```python
from build123d import *

# Parameters (mm, degrees)
SKETCH1_W           = 43.67
SKETCH1_H           = 21.69
SKETCH1_R           = 1.5
BOSS_EXTRUDE1_DEPTH = 1.5
SKETCH2_W           = 2.5
SKETCH2_H           = 2.5
BOSS_EXTRUDE2_DEPTH = 0.01
SKETCH3_W           = 2.5
SKETCH3_H           = 2.5
BOSS_EXTRUDE3_DEPTH = 0.01
SKETCH4_R           = 5
BOSS_EXTRUDE4_DEPTH = 12


with BuildPart() as part:
    # Sketch1 → Boss-Extrude1 (new body)
    with BuildSketch(Plane(origin=(0, 0, 0), x_dir=(1, 0, 0), z_dir=(0, 1, 0))):
        Rectangle(SKETCH1_W, SKETCH1_H)
        with Locations(Location((-15.145, 8.035, 0), (0, 0, 270))):
            Circle(SKETCH1_R, mode=Mode.SUBTRACT)
        with Locations(Location((15.095, -8.345, 0), (0, 0, 270))):
            Circle(SKETCH1_R, mode=Mode.SUBTRACT)
    extrude(amount=BOSS_EXTRUDE1_DEPTH)

    # Sketch2 → Boss-Extrude2 (add)
    with BuildSketch(Plane(origin=(0, 1.5, 0), x_dir=(1, 0, 0), z_dir=(0, 1, 0))):
        with Locations((-20.585, 9.595)):
            Rectangle(SKETCH2_W, SKETCH2_H)
        with Locations((-20.585, -9.595)):
            Rectangle(SKETCH2_W, SKETCH2_H)
    extrude(amount=BOSS_EXTRUDE2_DEPTH)

    # Sketch3 → Boss-Extrude3 (add)
    with BuildSketch(Plane(origin=(0, 1.5, 0), x_dir=(1, 0, 0), z_dir=(0, 1, 0))):
        with Locations((20.585, 9.595)):
            Rectangle(SKETCH3_W, SKETCH3_H)
        with Locations((20.585, -9.595)):
            Rectangle(SKETCH3_W, SKETCH3_H)
    extrude(amount=BOSS_EXTRUDE3_DEPTH)

    # Sketch4 → Boss-Extrude4 (add)
    with BuildSketch(Plane(origin=(0, 1.5, 0), x_dir=(1, 0, 0), z_dir=(0, 1, 0))):
        with Locations(Location((-12, 0, 0), (0, 0, 90))):
            Circle(SKETCH4_R)
        with Locations(Location((12, 0, 0), (0, 0, 90))):
            Circle(SKETCH4_R)
    extrude(amount=BOSS_EXTRUDE4_DEPTH)


solid = part.part
```
The listing builds one solid part. Answer for the finished solid, in the listing's coordinates (mm). A direction names the side the tool comes from. Coordinates: 2 decimals unless noted, no trailing zeros. Loops run counter-clockwise (first coordinate to the right, second up) from the corner with the lowest first, then second, coordinate; pieces in that order, holes last. Notation, with made-up numbers: M -35.5,21.5 L -28.5,21.5 A25 ccw -28.5,57.5 Z; hole C 87,76.5 d11. An arc over 180 degrees is marked long. Answer as a JSON object with one key per item and string values. Group by question number.
Item 1: Section C-C (y = 10.5) is taken. Write down the section's boundary in (x, z).
Item 2: Consider L1, parallel to Y at x = 11.5, z = 5.25; L2, parallel to X at y = 5.5, z = 2; L3, parallel to X at y = 1.75, z = 1.5. Determine where each line is inside the solid, lowest interval first.
Item 3: Section B-B (x = 12) is taken. Write down the section's boundary in (y, z) (3 decimals), and give its area (3 significant figures).
Item 4: Section A-A (z = 0) is taken. Write down the section's boundary in (x, y) (3 decimals), and give its area (3 significant figures).
Item 5: Which of the six approach directions +Z, -Z, +X, -X, +Y, -Y give full straight-line access (tool end or side, diameter ignored) to faces 4 (the face through (-21, 1.51, -10)), 5 (the face through (8, 7, -3))?
Item 6: Section D-D (x = 3) is taken. Write down the section's boundary in (y, z) (3 decimals).
Item 7: Determine the mould class of faces 1 (the face through (15.546, 0.74, 9.776)), 2 (the face through (-21.835, 1, 0)), 3 (the face through (21, 1.51, 10)) for opening direction X: +X half, -X half, draft (parallel to the pull), parting line (faces both ways), or undercut.
Item 8: Each of these flat-tipped pins is pushed along its axis until it touches: P1, Ø3, axis at x = -20, z = -10, coming from the +Y side; P2, Ø1.8, axis at x = 15.095, z = 8.345, coming from the +Y side. Where does it stop, or does it pass through?
Solved:
{
 "1": {"outline": "C -12,0 d10; C 12,0 d10"},
 "2": {"L1": "y = 0 to 1.5", "L2": "x = -16.58 to -7.42, 7.42 to 16.58", "L3": "x = -16.77 to -7.23, 7.23 to 16.77"},
 "3": {"outline": "M 0,-10.845 L 1.5,-10.845 L 1.5,-5 L 13.5,-5 L 13.5,5 L 1.5,5 L 1.5,10.845 L 0,10.845 Z", "area": "153 mm2"},
 "4": {"outline": "M -21.835,0 L 21.835,0 L 21.835,1.5 L 17,1.5 L 17,13.5 L 7,13.5 L 7,1.5 L -7,1.5 L -7,13.5 L -17,13.5 L -17,1.5 L -21.835,1.5 Z", "area": "306 mm2"},
 "5": {"face 4": "+Z, -Z, +X, -X, +Y", "face 5": "+Y"},
 "6": {"outline": "M 0,-10.845 L 1.5,-10.845 L 1.5,10.845 L 0,10.845 Z"},
 "7": {"face 1": "undercut", "face 2": "-X half", "face 3": "draft"},
 "8": {"P1": "stops at y = 1.51", "P2": "passes through"}
}
